Model file for the job. Use its own axes, mm. A direction names the side the tool comes from. Coordinates: 2 decimals unless noted, no trailing zeros. Order: outer loops, then holes, each group sorted by start corner. A loop starts at its lowest first (then second) coordinate and runs counter-clockwise, first axis right, second up.
from build123d import *

# Parameters (mm, degrees)
F9_W      = 185
F9_H      = 284.8
F10_DEPTH = 7.5
F11_W     = 200
F11_H     = 300
F12_DEPTH = 20
F16_R     = 70
F17_DEPTH = 157.5
F18_R     = 82.5
F19_DEPTH = 140
F20_R     = 35
F21_DEPTH = 157.5
F22_R     = 45
F23_DEPTH = 140
F13_W     = 40
F13_H     = 300
F24_DEPTH = 200
F25_SIZE  = 10
F26_SIZE2 = 9.99999
F26_SIZE  = 3.639692
F27_SIZE2 = 9.99999
F27_SIZE  = 3.639692


# Not quite as in the source:
# - a fillet or chamfer is up to 0.001 mm smaller than in the source, because OpenCascade refuses the exact size


with BuildPart() as f10:
    # F9 (on offset) → F10 (new body)
    with BuildSketch(Plane.XZ.offset(142.5)):
        with Locations((0, 150.1)):
            Rectangle(F9_W, F9_H)
    extrude(amount=F10_DEPTH)

    # F11 (on offset) → F12 (join)
    with BuildSketch(Plane.XZ.offset(150)):
        with Locations((0, 150)):
            Rectangle(F11_W, F11_H)
    extrude(amount=F12_DEPTH)

    # F16 (on offset) → F17 (cut, through all)
    with BuildSketch(Plane.XZ.offset(300)):
        with Locations((0, 100)):
            Circle(F16_R)
    extrude(amount=-F17_DEPTH, mode=Mode.SUBTRACT)

    # F18 (on offset) → F19 (cut, through all)
    with BuildSketch(Plane.XZ.offset(300)):
        with Locations((0, 100)):
            Circle(F18_R)
    extrude(amount=-F19_DEPTH, mode=Mode.SUBTRACT)

    # F20 (on offset) → F21 (cut, through all)
    with BuildSketch(Plane.XZ.offset(300)):
        with Locations((0, 238)):
            Circle(F20_R)
    extrude(amount=-F21_DEPTH, mode=Mode.SUBTRACT)

    # F22 (on offset) → F23 (cut, through all)
    with BuildSketch(Plane.XZ.offset(300)):
        with Locations((0, 238)):
            Circle(F22_R)
    extrude(amount=-F23_DEPTH, mode=Mode.SUBTRACT)

    # F13 (on offset) → F24 (cut, through all)
    with BuildSketch(Plane.YZ.offset(100)):
        with Locations((-200, 150)):
            Rectangle(F13_W, F13_H)
    extrude(amount=-F24_DEPTH, mode=Mode.SUBTRACT)

    # F25
    f25_edges = [f10.edges().sort_by_distance(p)[0] for p in [
        (100, -170, 150),
        (0, -170, 300),
        (-100, -170, 150),
        (0, -170, 0),
    ]]
    chamfer(f25_edges, length=F25_SIZE)

    # F26 (size 3.6397023427 and 10 in the source; OpenCascade refuses exactly that, so slightly less here)
    f26_edges = [f10.edges().sort_by_distance(p)[0] for p in [
        (-82.5, -170, 100),
    ]]
    f26_side = f10.faces().sort_by_distance((86.671337, -170, 150))[0]
    chamfer(f26_edges, length=F26_SIZE, length2=F26_SIZE2, reference=f26_side)

    # F27 (size 3.6397023427 and 10 in the source; OpenCascade refuses exactly that, so slightly less here)
    f27_edges = [f10.edges().sort_by_distance(p)[0] for p in [
        (-45, -170, 238),
    ]]
    f27_side = f10.faces().sort_by_distance((-89.468355, -170, 100))[0]
    chamfer(f27_edges, length=F27_SIZE, length2=F27_SIZE2, reference=f27_side)


solid = f10.part
Q1. Probe line 1 (Z direction, x = 0, y = -159.95); line 2 (Z direction, x = -20.5, y = -152.5); line 3 (Y direction, x = 14.5, z = 179.5). List the from-to ranges inside material, lowest first.
Established:
line 1: z = 0 to 30, 170 to 203, 273 to 300
line 2: z = 0 to 33.07, 166.93 to 209.63, 266.37 to 300
line 3: y = -160 to -142.5
Q2. Mould opens along Z. For faces 6 (the face through (-17.923, -160.486, 19.289)), 7 (the face through (-97, -150, 151)), 8 (the face through (-1, -165, 5)), 9 (the face through (23.1, -160, 211.5)) say: pulls with the +Z half, pulls with the -Z half, needs draft (parallel to the pull), parting line crosses it, or undercut.
Established:
face 6: undercut
face 7: needs draft
face 8: pulls with the -Z half
face 9: undercut
Q3. Drop flat-ended pins along their axis: P1, Ø2, axis at y = -148, z = 100, coming from the +X side; P2, Ø1.5, axis at x = -31, z = 174.5, coming from the -Y side; P3, Ø4, axis at x = 6, y = -147, coming from the +Z side. Give the stop position or say it passes through.
Established:
P1: stops at x = 92.5
P2: stops at y = -160
P3: stops at z = 292.5
Q4. Cut at C-C, the plane y = -154.5. List the corners of the cut face in (x, z).
Established:
outline: (-100, 0) - (100, 0) - (100, 300) - (-100, 300) - close; hole circle Ø140 at (0, 100); hole circle Ø70 at (0, 238)
Q5. Which spindle directions (+Z, -Z, +X, -X, +Y, -Y) get a long thin tool onto all of the face, cutting with end or side? Do faces 1 (the face through (-1, -146, 7.7)), 2 (the face through (-92.5, -146, 148)), 3 (the face through (24.287, -160.486, 276.093)), 4 (the face through (-1, -146, 292.5)), 5 (the face through (92.5, -146, 148)). Say none if no direction does.
Established:
face 1: -Z, +X, -X, +Y
face 2: +Z, -Z, -X, +Y
face 3: -Y
face 4: +Z, +X, -X, +Y
face 5: +Z, -Z, +X, +Y
Q6. Cut at A-A, the plane x = 0. Count the separate pieces of the cut face and the enclosed holes in it, plus the area to 3 significant figures.
Established:
separate pieces: 3
enclosed holes: 0
area: 1,740 mm2
